Here's how the part is built. I have some questions about the finished solid (model axes, mm). Give positions to 0.01 mm unless a question says otherwise; leave off trailing zeros. Loops run counter-clockwise (first coordinate to the right, second up) from the corner with the lowest first, then second, coordinate; pieces in that order, holes last. Notation, with made-up numbers: M 27,7 L 33,7 A8 cw 33,11 Z; hole C 2.5,66.5 d5. An arc over 180 degrees is marked long. Write item = value, one per line. Start each with the question number.
```python
from build123d import *

# Parameters (mm, degrees)
SKETCH1_W                   = 34
SKETCH1_H                   = 38
BASE_FLANGE1_DEPTH          = 2
TAP_DRILL_FOR_M3X0_5_TAP1_D = 2.5
CUT_EXTRUDE1_DEPTH          = 10
CUT_EXTRUDE1_DEPTH_BACK     = 10
FILLET2_R                   = 1
FILLET1_R                   = 3


# Sheet-metal steps are written as plain solids
with BuildPart() as part:
    # Sketch1 → Base-Flange1 (new body)
    with BuildSketch(Plane(origin=(0, 0, 0), x_dir=(1, 0, 0), z_dir=(0, 1, 0))):
        Rectangle(SKETCH1_W, SKETCH1_H)
    extrude(amount=-BASE_FLANGE1_DEPTH)

    # Tap Drill for M3x0.5 Tap1 (through all)
    with Locations(Plane(origin=(0, 0, 0), x_dir=(1, 0, 0), z_dir=(0, 1, 0))):
        with Locations((-9, -13), (-9, 13)):
            Hole(TAP_DRILL_FOR_M3X0_5_TAP1_D / 2)

    # Sketch14 → Cut-Extrude1 (cut, two sides: drawn at the far end of the back side and taken through both)
    with BuildSketch(Plane(origin=(0, -2, 0), x_dir=(-1, 0, 0), z_dir=(0, -1, 0)).offset(-CUT_EXTRUDE1_DEPTH_BACK)):
        Polygon((-9.5, 19), (-5, 19), (-5, -3), (-9.5, -3), (-9.5, 7), (-26.223726354, 7), (-26.223726354, 19), align=None)
    extrude(amount=CUT_EXTRUDE1_DEPTH + CUT_EXTRUDE1_DEPTH_BACK, mode=Mode.SUBTRACT)

    # Fillet2
    fillet2_edges = [part.edges().sort_by_distance(p)[0] for p in [
        (9.5, -1, -7),
        (9.5, -1, 3),
        (5, -1, 3),
    ]]
    fillet(fillet2_edges, radius=FILLET2_R)

    # Fillet1
    fillet1_edges = [part.edges().sort_by_distance(p)[0] for p in [
        (5, -1, -19),
        (17, -1, -7),
        (-17, -1, -19),
        (17, -1, 19),
        (-17, -1, 19),
    ]]
    fillet(fillet1_edges, radius=FILLET1_R)


solid = part.part
```
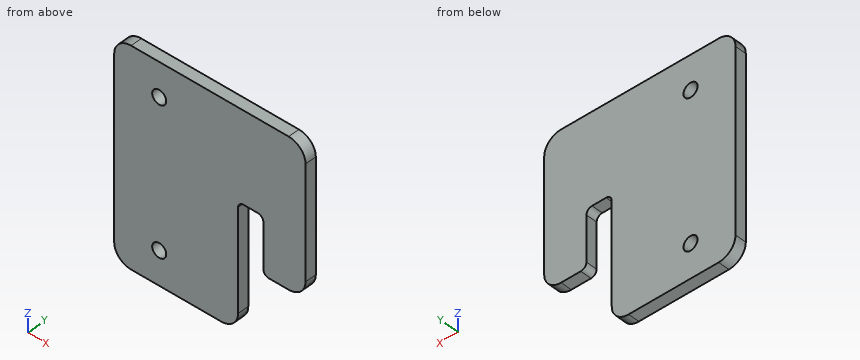
Q1. Will these pins go through, and if not, where does the flat tip stop? pin 1 (1 mm diameter, centred on x = 7.5, y = -1, fed in from -Z); pin 2 (0.6 mm diameter, centred on y = -1, z = -11.5, fed in from +X).
Q2. If we section it at C-C, the plane y = -1: List the corners of the cut face in (x, z) for me, then the cut area to 3 significant figures.
Q3. If I drill on line 1 along Z through (x, y) = (-9, -0.7); line 2 along X through (y, z) = (-0.9, 13); line 3 along X through (y, z) = (-1.2, -13), over which ranges is the centre line in solid material (lowest first)?
Q4. If we section it at D-D, the plane z = -1: List the corners of the cut face in (x, y) for me, then the cut area to 3 significant figures.
Q5. If we section it at B-B, the plane x = -9: List the corners of the cut face in (y, z) for me.
Q6. If we section it at A-A, the plane z = 13: List the corners of the cut face in (x, y) for me, then the cut area to 3 significant figures.
Resolved:
q1.pin_1 = 3
q1.pin_2 = 5
q2.outline = M -17,-16 A3 ccw -14,-19 L 2,-19 A3 ccw 5,-16 L 5,2 A1 cw 6,3 L 8.5,3 A1 cw 9.5,2 L 9.5,-6 A1 ccw 10.5,-7 L 14,-7 A3 ccw 17,-4 L 17,16 A3 ccw 14,19 L -14,19 A3 ccw -17,16 Z; hole C -9,-13 d2.5; hole C -9,13 d2.5
q2.area = 1,080 mm²
q3.line_1 = -19 to -14.25, -11.75 to 11.75, 14.25 to 19
q3.line_2 = -17 to -10.25, -7.75 to 17
q3.line_3 = -17 to -10.25, -7.75 to 5
q4.outline = M -17,-2 L 5,-2 L 5,0 L -17,0 Z; M 9.5,-2 L 17,-2 L 17,0 L 9.5,0 Z
q4.area = 59.0 mm²
q5.outline = M -2,-19 L 0,-19 L 0,-14.25 L -2,-14.25 Z; M -2,-11.75 L 0,-11.75 L 0,11.75 L -2,11.75 Z; M -2,14.25 L 0,14.25 L 0,19 L -2,19 Z
q6.outline = M -17,-2 L -10.25,-2 L -10.25,0 L -17,0 Z; M -7.75,-2 L 17,-2 L 17,0 L -7.75,0 Z
q6.area = 63.0 mm²
